Could you check a few things on this model? Use its own coordinates, in mm. Face numbers are marked on the shaded views. A direction names the side the tool comes from. Give positions to 0.01 mm unless a question says otherwise; leave off trailing zeros. Order: outer loops, then holes, each group sorted by start corner. A loop starts at its lowest first (then second) coordinate and runs counter-clockwise, first axis right, second up. Notation, with made-up numbers: M 30,59 L 52,59 A21 ccw 52,97 Z; hole C -16,74 d3. An arc over 180 degrees is marked long. Return JSON: item names as keys, results as strings. Group by question number.
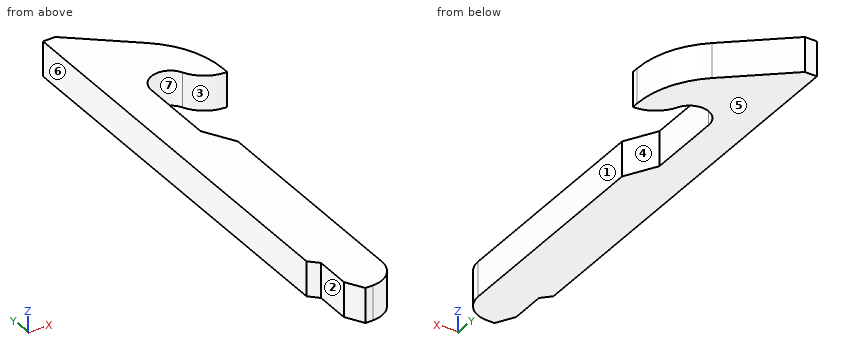
```python
from build123d import *

# Parameters (mm, degrees)
BOSS_EXTRUDE1_DEPTH = 10


with BuildPart() as part:
    # Sketch1 → Boss-Extrude1 (new, symmetric)
    with BuildSketch(Plane.XY):
        with BuildLine():
            Line((5, 10), (10.773502692, 0))
            Line((10.773502692, 0), (15, 0))
            ThreePointArc((15, 0), (25.606601718, 4.393398282), (30, 15))
            Line((30, 15), (30, 140.679491924))
            Line((30, 140.679491924), (20, 158))
            Line((20, 158), (20, 201))
            ThreePointArc((20, 201), (28.580322602, 211.73057134), (40.935483871, 205.720821989))
            ThreePointArc((40.935483871, 205.720821989), (48.315110065, 197.397534592), (59, 194.304134696))
            Line((59, 194.304134696), (59, 198))
            ThreePointArc((59, 198), (54.324714747, 219.11090318), (41.173190677, 236.273826587))
            Line((41.173190677, 236.273826587), (7, 265))
            Line((7, 265), (0, 265))
            Line((0, 265), (0, 35))
            Line((0, 35), (5, 30))
            Line((5, 30), (5, 10))
        make_face()
    extrude(amount=BOSS_EXTRUDE1_DEPTH, both=True)


solid = part.part
```
1. If we mould it in two halves opening along X, with no side actions, what happens to the marked faces 5, 6 and 7? For each: pulls with the +X half, pulls with the -X half, needs draft (parallel to the pull), parting line crosses it, or undercut.
2. Which directions (+Z, -Z, +X, -X, +Y, -Y) give clear straight access to the entire face, cutting with the end or side of a thin tool? Please do the marked faces 1, 2, 3 and 4.
3. For pin 1 (6 mm diameter, centred on y = 21, z = 1, fed in from -X); pin 2 (6 mm diameter, centred on y = 174.5, z = 2.5, fed in from +X); pin 3 (2 mm diameter, centred on x = 21.5, z = 7, fed in from +Y), each with a flat end and sliding along its axis, tell me the tip position at first contact or that it passes through.
4. Imagine slicing it at C-C, the plane x = 37. Please give me the cut outline in (y, z).
5. I need wall thicknesses on L1, parallel to X at y = 135, z = 7; L2, parallel to X at y = 170.5, z = 5; L3, parallel to Y at x = 26, z = 5.25. Which ranges of each line are inside material? Lowest first, please. Write a range as from..to.
6. Imagine slicing it at A-A, the plane z = -1.75. Please give me the cut outline in (x, y), plus the area to 3 significant figures.
7. Imagine slicing it at B-B, the plane y = 56. Please give me the cut outline in (x, z).
Values:
{
 "1": {"face 5": "needs draft", "face 6": "pulls with the -X half", "face 7": "undercut"},
 "2": {"face 1": "+Z, -Z, +X, -Y", "face 2": "+Z, -Z, -X, -Y", "face 3": "+Z, -Z, -Y", "face 4": "+Z, -Z, +X"},
 "3": {"pin 1": "stops at x = 5", "pin 2": "stops at x = 20", "pin 3": "stops at y = 253.65"},
 "4": {"outline": "M 210.22,-10 L 239.78,-10 L 239.78,10 L 210.22,10 Z"},
 "5": {"L1": "x = 0..30", "L2": "x = 0..20", "L3": "y = 4.8..147.61, 210.8..249.03"},
 "6": {"outline": "M 0,35 L 5,30 L 5,10 L 10.77,0 L 15,0 A15 ccw 30,15 L 30,140.68 L 20,158 L 20,201 A11 cw 40.94,205.72 A20 ccw 59,194.3 L 59,198 A50 ccw 41.17,236.27 L 7,265 L 0,265 Z", "area": "7,710 mm²"},
 "7": {"outline": "M 0,-10 L 30,-10 L 30,10 L 0,10 Z"}
}
